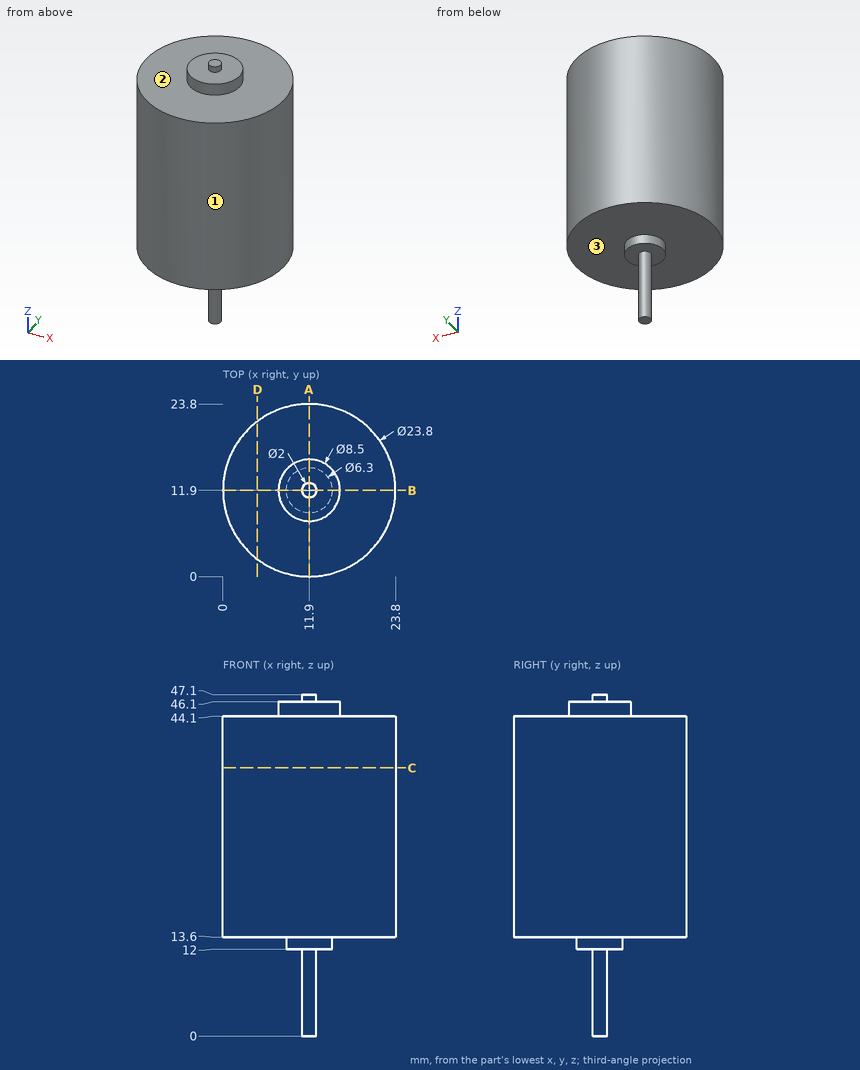
Input: dimensioned drawing with shaded views. Units: mm. Origin: part minimum x, y, z. A direction names the side the tool comes from. Coordinates: 2 decimals unless noted, no trailing zeros. Order: outer loops, then holes, each group sorted by start corner. A loop starts at its lowest first (then second) coordinate and runs counter-clockwise, first axis right, second up. Notation, with made-up numbers: M 48.25,34.25 L 59.25,34.25 A34 ccw 59.25,65.25 Z; hole C 45,79 d10. An arc over 180 degrees is marked long. Write each question's results on one line, items separated by ' | '. Start each with the question number.
Item 1: First-contact query: pin 1 Ø5 at (x, z) = (20.5, 30.5) entering from -Y; pin 2 Ø6 at (x, y) = (13.5, 16) entering from +Z; pin 3 Ø5 at (x, y) = (8, 4) entering from +Z. Flat tips, straight axial feed; report the tip coordinate or a pass-through.
Item 2: Cut plane D-D (x = 4.75). Return loops of the section in (y, z).
Item 3: Set-up query: the marked faces 1, 2 and 3. Return all of +Z, -Z, +X, -X, +Y, -Y with unobstructed straight access to the full face (end or side cutting, diameter ignored); none if empty.
Item 4: Line query: probe 1 along Z at (x, y) = (8.5, 10); probe 2 along Z at (x, y) = (15.25, 17.5); probe 3 along Y at (x, z) = (14, 33). Output: solid intervals per line, ascending.
Item 5: Cut plane A-A (x = 11.9). Return loops of the section in (y, z), and give its area (3 significant figures).
Item 6: Cut plane C-C (z = 37). Return loops of the section in (x, y).
Checked values:
1) pin 1: stops at y = 1.68 | pin 2: stops at z = 46.1 | pin 3: stops at z = 44.1
2) outline: M 2.39,13.6 L 21.41,13.6 L 21.41,44.1 L 2.39,44.1 Z
3) face 1: +Z, -Z | face 2: +Z | face 3: -Z
4) probe 1: z = 13.6 to 46.1 | probe 2: z = 13.6 to 44.1 | probe 3: y = 0.19 to 23.61
5) outline: M 0,13.6 L 8.75,13.6 L 8.75,12 L 10.9,12 L 10.9,0 L 12.9,0 L 12.9,12 L 15.05,12 L 15.05,13.6 L 23.8,13.6 L 23.8,44.1 L 16.15,44.1 L 16.15,46.1 L 12.9,46.1 L 12.9,47.1 L 10.9,47.1 L 10.9,46.1 L 7.65,46.1 L 7.65,44.1 L 0,44.1 Z | area: 779 mm2
6) outline: C 11.9,11.9 d23.8
